from build123d import *

# Parameters (mm, degrees)
SKETCH1_W           = 350
SKETCH1_H           = 56.2
BOSS_EXTRUDE1_DEPTH = 10
SKETCH2_W           = 56.2
SKETCH2_H           = 56.2
CUT_EXTRUDE1_DEPTH  = 5
SKETCH3_W           = 10
SKETCH3_H           = 56.2
BOSS_EXTRUDE2_DEPTH = 10
SKETCH4_W           = 10
SKETCH4_H           = 56.2
BOSS_EXTRUDE3_DEPTH = 10
CUT_EXTRUDE2_DEPTH  = 56.2
SKETCH6_W           = 10
SKETCH6_H           = 56.2
BOSS_EXTRUDE4_DEPTH = 10
SKETCH7_W           = 10
SKETCH7_H           = 56.2
BOSS_EXTRUDE5_DEPTH = 10
CUT_EXTRUDE3_DEPTH  = 56.2
SKETCH9_W           = 30
SKETCH9_H           = 30
CUT_EXTRUDE4_DEPTH  = 5
SKETCH10_R          = 3
CUT_EXTRUDE5_DEPTH  = 5
SKETCH11_W          = 2.5
SKETCH11_H          = 15
CUT_EXTRUDE6_DEPTH  = 7
SKETCH12_W          = 2.5
SKETCH12_H          = 15
CUT_EXTRUDE8_DEPTH  = 7
SKETCH14_W          = 56.2
SKETCH14_H          = 56.2
SKETCH14_R          = 3
SKETCH14_W_2        = 30
SKETCH14_H_2        = 30
BOSS_EXTRUDE7_DEPTH = 5
SKETCH15_W          = 56.2
SKETCH15_H          = 56.2
CUT_EXTRUDE9_DEPTH  = 5


with BuildPart() as part:
    # Sketch1 → Boss-Extrude1 (new body)
    with BuildSketch(Plane.XY):
        Rectangle(SKETCH1_W, SKETCH1_H)
    extrude(amount=BOSS_EXTRUDE1_DEPTH)

    # Sketch2 → Cut-Extrude1 (cut)
    with BuildSketch(Plane.XY.offset(10)):
        Rectangle(SKETCH2_W, SKETCH2_H)
    extrude(amount=-CUT_EXTRUDE1_DEPTH, mode=Mode.SUBTRACT)

    # Sketch3 → Boss-Extrude2 (add)
    with BuildSketch(Plane(origin=(175, 0, 0), x_dir=(0, 0, -1), z_dir=(1, 0, 0))):
        with Locations((-5, 0)):
            Rectangle(SKETCH3_W, SKETCH3_H)
    extrude(amount=BOSS_EXTRUDE2_DEPTH)

    # Sketch4 → Boss-Extrude3 (add)
    with BuildSketch(Plane.XY.offset(10)):
        with Locations((180, 0)):
            Rectangle(SKETCH4_W, SKETCH4_H)
    extrude(amount=BOSS_EXTRUDE3_DEPTH)

    # Sketch5 → Cut-Extrude2 (cut)
    with BuildSketch(Plane(origin=(0, 28.1, 0), x_dir=(1, 0, 0), z_dir=(0, 1, 0))):
        Polygon((175, -20), (185, -10), (185, -20), align=None)
    extrude(amount=-CUT_EXTRUDE2_DEPTH, mode=Mode.SUBTRACT)

    # Sketch6 → Boss-Extrude4 (add)
    with BuildSketch(Plane.ZY.offset(175)):
        with Locations((5, 0)):
            Rectangle(SKETCH6_W, SKETCH6_H)
    extrude(amount=BOSS_EXTRUDE4_DEPTH)

    # Sketch7 → Boss-Extrude5 (add)
    with BuildSketch(Plane.XY.offset(10)):
        with Locations((-180, 0)):
            Rectangle(SKETCH7_W, SKETCH7_H)
    extrude(amount=BOSS_EXTRUDE5_DEPTH)

    # Sketch8 → Cut-Extrude3 (cut)
    with BuildSketch(Plane(origin=(0, 28.1, 0), x_dir=(1, 0, 0), z_dir=(0, 1, 0))):
        Polygon((-175, -20), (-185, -10), (-185, -20), align=None)
    extrude(amount=-CUT_EXTRUDE3_DEPTH, mode=Mode.SUBTRACT)

    # Sketch9 → Cut-Extrude4 (cut)
    with BuildSketch(Plane.XY.offset(5)):
        Rectangle(SKETCH9_W, SKETCH9_H)
    extrude(amount=-CUT_EXTRUDE4_DEPTH, mode=Mode.SUBTRACT)

    # Sketch10 → Cut-Extrude5 (cut)
    with BuildSketch(Plane.XY.offset(5)):
        with Locations((21.55, 21.55)):
            Circle(SKETCH10_R)
        with Locations((-21.55, -21.55)):
            Circle(SKETCH10_R)
        with Locations((-21.55, 21.55)):
            Circle(SKETCH10_R)
        with Locations((21.55, -21.55)):
            Circle(SKETCH10_R)
    extrude(amount=-CUT_EXTRUDE5_DEPTH, mode=Mode.SUBTRACT)

    # Sketch11 → Cut-Extrude6 (cut)
    with BuildSketch(Plane(origin=(97.5, 0, 97.5), x_dir=(0.707106781, 0, -0.707106781), z_dir=(0.707106781, 0, 0.707106781))):
        with Locations((116.672618896, 0)):
            Rectangle(SKETCH11_W, SKETCH11_H)
    extrude(amount=-CUT_EXTRUDE6_DEPTH, mode=Mode.SUBTRACT)

    # Sketch12 → Cut-Extrude8 (cut)
    with BuildSketch(Plane(origin=(-97.5, 0, 97.5), x_dir=(0.707106781, 0, 0.707106781), z_dir=(-0.707106781, 0, 0.707106781))):
        with Locations((-116.672618896, 0)):
            Rectangle(SKETCH12_W, SKETCH12_H)
    extrude(amount=-CUT_EXTRUDE8_DEPTH, mode=Mode.SUBTRACT)

    # Sketch14 → Boss-Extrude7 (add)
    with BuildSketch(Plane.XY.offset(5)):
        Rectangle(SKETCH14_W, SKETCH14_H)
        with Locations((-21.55, 21.55)):
            Circle(SKETCH14_R, mode=Mode.SUBTRACT)
        with Locations((21.55, 21.55)):
            Circle(SKETCH14_R, mode=Mode.SUBTRACT)
        with Locations((21.55, -21.55)):
            Circle(SKETCH14_R, mode=Mode.SUBTRACT)
        with Locations((-21.55, -21.55)):
            Circle(SKETCH14_R, mode=Mode.SUBTRACT)
        Rectangle(SKETCH14_W_2, SKETCH14_H_2, mode=Mode.SUBTRACT)
    extrude(amount=BOSS_EXTRUDE7_DEPTH)

    # Sketch15 → Cut-Extrude9 (cut)
    with BuildSketch(Plane(origin=(0, 0, 0), x_dir=(-1, 0, 0), z_dir=(0, 0, -1))):
        Rectangle(SKETCH15_W, SKETCH15_H)
    extrude(amount=-CUT_EXTRUDE9_DEPTH, mode=Mode.SUBTRACT)


solid = part.part
Verification items for the finished model (mm, model axes). A direction names the side the tool comes from. Give positions to 0.01 mm unless a question says otherwise; leave off trailing zeros. Write each loop counter-clockwise with the first axis right and the second up, starting at its lowest first coordinate (ties: lowest second). Pieces come first, ordered by that corner, then holes. Notation, with made-up numbers: M 6,79 L 33,79 A12 ccw 33,87 Z; hole C 8.5,69.5 d3. An arc over 180 degrees is marked long. Put each result on its own line as item: value. Start each with the question number.
1. Section check D-D (x = -104.5). Record the cut outline in (y, z), and give its area (3 significant figures).
2. Section check B-B (x = -21.55). Record the cut outline in (y, z).
3. Set-up check for faces 1 (the face through (-2.6, 28.1, 5.4)), 2 (the face through (175, 0, 15)), 3 (the face through (108, 0, 0)), 4 (the face through (19, 0, 5)), 5 (the face through (-178, 7.5, 13)): record each of +Z, -Z, +X, -X, +Y, -Y from which the full face is reachable in a straight line by a thin tool's end or side.
4. Section check C-C (y = -21.55). Record the cut outline in (x, z), and give its area (3 significant figures).
5. Section check A-A (y = 1.5). Record the cut outline in (x, z), and give its area (3 significant figures).
6. Scan lines: line 1 along X through (y, z) = (21.55, 8.5); line 2 along Y through (x, z) = (-21.55, 7.3); line 3 along X through (y, z) = (11, 9.25). Record each from-to range of solid material in increasing order. Write a range as [from, to].
7. Go/stop test with flat-tipped pins: pin 1 Ø8 at (x, y) = (-65.5, 14.5) entering from +Z; pin 2 Ø8 at (y, z) = (-4.5, 16) entering from -X; pin 3 Ø5 at (y, z) = (-2, 17) entering from +X. Record where each tip stops, or that it passes through.
8. Draft check along Z on faces 6 (the face through (-178, -7.5, 13)), 7 (the face through (-2.6, -28.1, 5.4)), 8 (the face through (179, 0, 16)), 9 (the face through (178, -7.5, 13)). Enter one of: +Z half, -Z half, draft (parallel to the pull), parting line (faces both ways), or undercut.
Answer list:
1. outline: M -28.1,0 L 28.1,0 L 28.1,10 L -28.1,10 Z
1. area: 562 mm2
2. outline: M -28.1,5 L -24.55,5 L -24.55,10 L -28.1,10 Z; M -18.55,5 L 18.55,5 L 18.55,10 L -18.55,10 Z; M 24.55,5 L 28.1,5 L 28.1,10 L 24.55,10 Z
3. face 1: +Z, -Z, +X, -X, +Y
3. face 2: +Z, +Y, -Y
3. face 3: -Z, +X, -X, +Y, -Y
3. face 4: -Z, +Y, -Y
3. face 5: none
4. outline: M -185,0 L -28.1,0 L -28.1,5 L -24.55,5 L -24.55,10 L -175,10 L -175,20 L -185,10 Z; M -18.55,5 L 18.55,5 L 18.55,10 L -18.55,10 Z; M 24.55,5 L 28.1,5 L 28.1,0 L 185,0 L 185,10 L 175,20 L 175,10 L 24.55,10 Z
4. area: 3,460 mm2
5. outline: M -185,0 L -28.1,0 L -28.1,5 L -15,5 L -15,10 L -175,10 L -175,10.1 L -175.93,9.17 L -180.88,14.12 L -185,10 Z; M -179.12,15.88 L -175,11.77 L -175,20 Z; M 15,5 L 28.1,5 L 28.1,0 L 185,0 L 185,10 L 180.88,14.12 L 175.93,9.17 L 175,10.1 L 175,10 L 15,10 Z; M 175,11.77 L 179.12,15.88 L 175,20 Z
5. area: 3,340 mm2
6. line 1: [-185, -24.55], [-18.55, 18.55], [24.55, 185]
6. line 2: [-28.1, -24.55], [-18.55, 18.55], [24.55, 28.1]
6. line 3: [-185, -15], [15, 185]
7. pin 1: z = 10
7. pin 2: x = -183
7. pin 3: x = 179.12
8. face 6: undercut
8. face 7: draft
8. face 8: +Z half
8. face 9: undercut
